Geometry check sheet. Reference: the model listing, model coordinates, mm. A direction names the side the tool comes from. Coordinates: 2 decimals unless noted, no trailing zeros. Write each loop counter-clockwise with the first axis right and the second up, starting at its lowest first coordinate (ties: lowest second). Pieces come first, ordered by that corner, then holes. Notation, with made-up numbers: (88, -39) -> (111, -39) arc R25 ccw to (111, -11) -> close; hole circle Ø1 at (61, 84). An arc over 180 degrees is marked (long way). Use a Markdown table: item, result.
```python
from build123d import *

# Parameters (mm, degrees)
SKETCH1_R           = 2.3
BOSS_EXTRUDE2_DEPTH = 12
CUT_EXTRUDE1_DEPTH  = 10.5
BOSS_EXTRUDE3_START = -1.5
SKETCH4_W           = 22
SKETCH4_H           = 1
BOSS_EXTRUDE3_DEPTH = 12
SKETCH5_W           = 12
SKETCH5_H           = 56
CUT_EXTRUDE2_DEPTH  = 10.5


with BuildPart() as part:
    # Sketch1 → Boss-Extrude2 (new body)
    with BuildSketch(Plane(origin=(0, 0, 0), x_dir=(1, 0, 0), z_dir=(0, 1, 0))):
        Polygon((12, 27), (12, -27), (10, -27), (-10, -27), (-10, -20), (-10, 20), (-10, 27), (10, 27), align=None)
        with Locations(Location((-5.76, 24.37, 0), (0, 0, 270))):
            Circle(SKETCH1_R, mode=Mode.SUBTRACT)
        with Locations(Location((-5.76, -24.37, 0), (0, 0, 270))):
            Circle(SKETCH1_R, mode=Mode.SUBTRACT)
    extrude(amount=BOSS_EXTRUDE2_DEPTH)

    # Sketch3 → Cut-Extrude1 (cut)
    with BuildSketch(Plane.XZ):
        Polygon((10, 27), (-2, 27), (-2, 21), (-10, 21), (-10, -21), (-2, -21), (-2, -27), (10, -27), align=None)
    extrude(amount=-CUT_EXTRUDE1_DEPTH, mode=Mode.SUBTRACT)

    # Sketch4 → Boss-Extrude3 (add)
    with BuildSketch(Plane.XZ.offset(-10.5).offset(BOSS_EXTRUDE3_START)):
        with Locations((1, 27.5)):
            Rectangle(SKETCH4_W, SKETCH4_H)
        with Locations((1, -27.5)):
            Rectangle(SKETCH4_W, SKETCH4_H)
    extrude(amount=BOSS_EXTRUDE3_DEPTH)

    # Sketch5 → Cut-Extrude2 (cut)
    with BuildSketch(Plane.XZ.offset(-10.5)):
        with Locations((4, 0)):
            Rectangle(SKETCH5_W, SKETCH5_H)
    extrude(amount=CUT_EXTRUDE2_DEPTH, mode=Mode.SUBTRACT)


solid = part.part
```
Item 1: Depth check by flat-ended pin: P1, Ø6, axis at x = 0, z = -9, coming from the -Y side. Enter the tip coordinate at first touch or a pass-through.
Answer block:
| item | result |
|---|---|
| P1 | stops at y = 10.5 |
Item 2: Tool access check on faces 4 (the flat face through (-6, 5, -21)), 5 (the flat face through (10, 5, 0)), 6 (the flat face through (11, 0, 0)). Record the directions out of +Z, -Z, +X, -X, +Y, -Y that give a thin tool (end or side, any length) a straight path to the whole face; none if there is none.
Answer block:
| item | result |
|---|---|
| face 4 | -X, -Y |
| face 5 | +Z, -Z, -Y |
| face 6 | +Z, -Z, +X, -X, -Y |
Item 3: Thickness scan on L1, parallel to X at y = 8.25, z = 24.37; L2, parallel to Z at x = -4.5, y = 11.5; L3, parallel to Z at x = -7.5, y = 9.25. Record the ranges inside material, lowest first. Write a range as [from, to].
Answer block:
| item | result |
|---|---|
| L1 | x = [-10, -8.06], [-3.46, -2], [10, 12] |
| L2 | z = [-28, -26.29], [-22.45, 22.45], [26.29, 28] |
| L3 | z = [-28, -25.87], [-22.87, -21], [21, 22.87], [25.87, 28] |
Item 4: Section check A-A on y = 5. Record the boundary of the cut face in (x, z), then the cut area to 3 significant figures.
Answer block:
| item | result |
|---|---|
| outline | (-10, -28) -> (-2, -28) -> (-2, -21) -> (-10, -21) -> close; (-10, 21) -> (-2, 21) -> (-2, 28) -> (-10, 28) -> close; (10, -28) -> (12, -28) -> (12, 28) -> (10, 28) -> close; hole circle Ø4.6 at (-5.76, -24.37); hole circle Ø4.6 at (-5.76, 24.37) |
| area | 191 mm^2 |
Item 5: Section check B-B on z = -24.37. Record the boundary of the cut face in (x, y).
Answer block:
| item | result |
|---|---|
| outline | (-10, 0) -> (-8.06, 0) -> (-8.06, 12) -> (-10, 12) -> close; (-3.46, 0) -> (-2, 0) -> (-2, 10.5) -> (10, 10.5) -> (10, 0) -> (12, 0) -> (12, 12) -> (-3.46, 12) -> close |
Item 6: Section check C-C on x = -5.76. Record the boundary of the cut face in (y, z), then the cut area to 3 significant figures.
Answer block:
| item | result |
|---|---|
| outline | (0, -28) -> (12, -28) -> (12, -26.67) -> (0, -26.67) -> close; (0, -22.07) -> (12, -22.07) -> (12, 22.07) -> (0, 22.07) -> (0, 21) -> (10.5, 21) -> (10.5, -21) -> (0, -21) -> close; (0, 26.67) -> (12, 26.67) -> (12, 28) -> (0, 28) -> close |
| area | 121 mm^2 |
Item 7: Mould release check, pull along Z, two halves, no side actions. Record for faces 1 (the flat face through (-2, 5, 24)), 2 (the cylindrical face through (-6.641, 5.916, 26.495)), 3 (the flat face through (-4, 6, -28)): +Z half, -Z half, draft (parallel to the pull), parting line (faces both ways), or undercut.
Answer block:
| item | result |
|---|---|
| face 1 | draft |
| face 2 | undercut |
| face 3 | -Z half |
Item 8: Section check D-D on y = 11. Record the boundary of the cut face in (x, z), then the cut area to 3 significant figures.
Answer block:
| item | result |
|---|---|
| outline | (-10, -28) -> (12, -28) -> (12, 28) -> (-10, 28) -> close; hole circle Ø4.6 at (-5.76, -24.37); hole circle Ø4.6 at (-5.76, 24.37) |
| area | 1,200 mm^2 |
